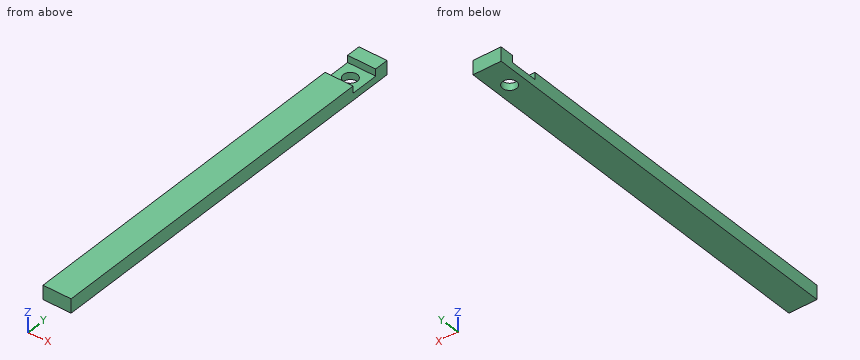
```python
from build123d import *

# Parameters (mm, degrees)
SKETCH1_W           = 25.4
SKETCH1_H           = 12.7
BOSS_EXTRUDE1_DEPTH = 355.6
SKETCH2_W           = 6.35
SKETCH2_H           = 25.4
CUT_EXTRUDE1_DEPTH  = 357.732126392
SKETCH3_R           = 6.35
CUT_EXTRUDE2_DEPTH  = 357.562536591


with BuildPart() as part:
    # Sketch1 → Boss-Extrude1 (new body)
    with BuildSketch(Plane(origin=(0, 0, 0), x_dir=(1, 0, 0), z_dir=(0, 1, 0))):
        with Locations((12.7, 6.35)):
            Rectangle(SKETCH1_W, SKETCH1_H)
    extrude(amount=BOSS_EXTRUDE1_DEPTH)

    # Sketch2 → Cut-Extrude1 (cut, through all)
    with BuildSketch(Plane(origin=(25.4, 0, 0), x_dir=(0, 0, -1), z_dir=(1, 0, 0))):
        with Locations((3.175, 330.2)):
            Rectangle(SKETCH2_W, SKETCH2_H)
    extrude(amount=-CUT_EXTRUDE1_DEPTH, mode=Mode.SUBTRACT)

    # Sketch3 → Cut-Extrude2 (cut, through all)
    with BuildSketch(Plane.XY.offset(-6.35)):
        with Locations((12.7, 330.2)):
            Circle(SKETCH3_R)
    extrude(amount=-CUT_EXTRUDE2_DEPTH, mode=Mode.SUBTRACT)


solid = part.part
```
Geometry check sheet. Reference: the model listing, model coordinates, mm. Coordinates: 2 decimals unless noted, no trailing zeros. Write each loop counter-clockwise with the first axis right and the second up, starting at its lowest first coordinate (ties: lowest second). Pieces come first, ordered by that corner, then holes. Notation, with made-up numbers: M 10,28.25 L 52,28.25 A13 ccw 52,49.25 Z; hole C 59,77 d10. An arc over 180 degrees is marked long. One line per item, written item: value. Start each with the question number.
(1) Sectioned sample at A-A, the plane y = 330.2. Enter the section's corners in (x, z).
(2) Scan lines: line 1 along Y through (x, z) = (16.75, -4.25); line 2 along X through (y, z) = (330.2, -9.75); line 3 along Y through (x, z) = (12.7, -7.25). Record each from-to range of solid material in increasing order. Write a range as [from, to].
(3) Depth check by flat-ended pin: pin 1 (7.5 mm diameter, centred on x = 15.5, y = 329, fed in from +Z). Enter the tip coordinate at first touch or a pass-through.
(4) Sectioned sample at B-B, the plane x = 12.7. Enter the section's corners in (y, z), and give its area (3 significant figures).
Filled sheet:
1. outline: M 0,-12.7 L 6.35,-12.7 L 6.35,-6.35 L 0,-6.35 Z; M 19.05,-12.7 L 25.4,-12.7 L 25.4,-6.35 L 19.05,-6.35 Z
2. line 1: [0, 317.5], [342.9, 355.6]
2. line 2: [0, 6.35], [19.05, 25.4]
2. line 3: [0, 323.85], [336.55, 355.6]
3. pin 1: z = -6.35
4. outline: M 0,-12.7 L 323.85,-12.7 L 323.85,-6.35 L 317.5,-6.35 L 317.5,0 L 0,0 Z; M 336.55,-12.7 L 355.6,-12.7 L 355.6,0 L 342.9,0 L 342.9,-6.35 L 336.55,-6.35 Z
4. area: 4,270 mm²
